Geometry check sheet. Reference: the model listing, model coordinates, mm. Face numbers are marked on the shaded views. A direction names the side the tool comes from. Coordinates: 2 decimals unless noted, no trailing zeros. Write each loop counter-clockwise with the first axis right and the second up, starting at its lowest first coordinate (ties: lowest second). Pieces come first, ordered by that corner, then holes. Notation, with made-up numbers: (33.25, 20) -> (42.25, 20) arc R27 cw to (42.25, 51) -> close; hole circle Ø5 at (74.25, 17.5). An arc over 180 degrees is marked (long way). One line per question, with ' | ' between items.
Autodesk Inventor part; units mm, degrees
ref_plane "YZ Plane" through (0, 0, 0) normal (1, 0, 0) x (0, 1, 0)
ref_plane "XZ Plane" through (0, 0, 0) normal (0, 1, 0) x (-1, 0, 0)
ref_plane "XY Plane" through (0, 0, 0) normal (0, 0, 1) x (1, 0, 0)
sketch "スケッチ1" plane through (0, 0, 0) normal (0, 1, 0) x (-1, 0, 0)
  circle A0 centre (0, 0) radius 27.5
  line L0 (13, 12.85) -> (-13, 12.85)
  line L1 (-13, 12.85) -> (-13, -12.85)
  line L2 (-13, -12.85) -> (13, -12.85)
  line L3 (13, -12.85) -> (13, 12.85)
  circle A1 centre (0, 0) radius 32.5
  circle A2 centre (0, 0) radius 36.5
  line L4 (0, 0) -> (18.4986, -32.0406)
  line L5 (0, 0) -> (31.6099, -18.25)
  line L6 (-13, -12.85) -> (0.651, -36.4942)
  line L7 (13.2, 12.8507) -> (13.2, -12.85)
  line L8 (13.2, -12.85) -> (13, -12.85)
  point P0 (13, 0)
  point P1 (0, 12.85)
  point P2 (13, -34.1065)
  point P3 (-13, -34.1065)
  point P4 (28.1458, -16.25)
  point P5 (13, -7.5056)
  point P6 (18.25, -31.6099)
  point P7 (16.25, -28.1458)
  point P8 (23.8157, -13.75)
  point P9 (-4.7839, -27.0807)
  point P10 (-1.6802, -32.4565)
  point P11 (13.2, -7.621)
  dimension "d0" = 55
  dimension "d1" = 12.85
  dimension "d2" = 26
  dimension "d3" = 5
  dimension "d4" = 4
  dimension "d11" = 60
  dimension "d12" = 30
  dimension "d16" = 0.2
extrude "押し出し1" add sketch "スケッチ1" along normal blind 4 contours L6 L2 L4 A0 | A0 L4 A1 L6 | L5 A1 L4 A0 | A0 L4 L2 L8 L7 L5 | A1 L4 A2 L6 | L5 A2 L4 A1
extrude "押し出し2" add sketch "スケッチ1" along normal blind 9.2 contours A0 L4 A1 L6 | L5 A1 L4 A0
extrude "押し出し3" add sketch "スケッチ1" along normal blind 14.8 contours A1 L4 A2 L6 | L5 A2 L4 A1
chamfer "面取り1" distance 8 angle 45 1 edges at (-18.5312, 0, -31.4459)
sketch "スケッチ2" plane through (-13.2, 0, -12.85) normal (0, 0, 1) x (1, 0, 0)
  circle A0 centre (21.2, 2) radius 0.8
  circle A1 centre (5.2, 2) radius 0.8
  point P0 (13.2, 0)
extrude "押し出し4" cut sketch "スケッチ2" against normal through all
sketch "スケッチ4" plane through (0, 14.8, 0) normal (0, 1, 0) x (1, 0, 0)
  circle A0 centre (-24.3952, 24.3952) radius 0.8
  line L0 (4.7839, 27.0807) -> (-0.651, 36.4942)
  arc A1 (-0.651, 36.4942) -> (-31.6099, 18.25) centre (0, 0) ccw
  line L1 (-31.6099, 18.25) -> (-23.8157, 13.75)
  arc A2 (4.7839, 27.0807) -> (-23.8157, 13.75) centre (0, 0) ccw
  circle A3 centre (-17.25, 29.8779) radius 0.8
  circle A4 centre (-8.9293, 33.3244) radius 0.8
  circle A5 centre (-24.3952, 24.3952) radius 0.8
extrude "押し出し6" cut sketch "スケッチ4" against normal blind 4 contours A0 | A3 | A4
properties part number "waist_side"
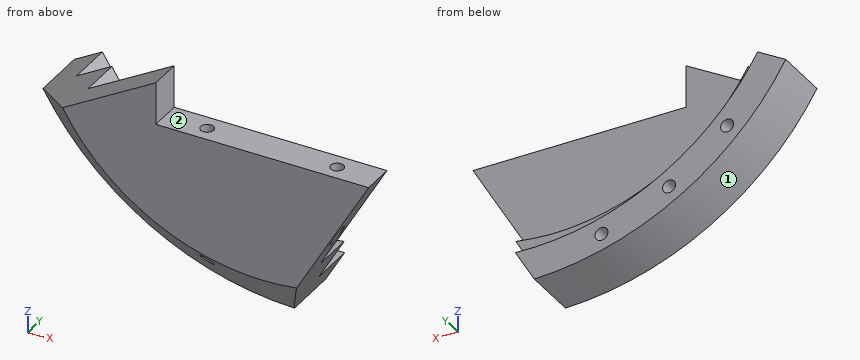
(1) Cross-section at A-A (y = 2). Record the cut outline in (x, z), plus the area to 3 significant figures.
Answers below:
outline: (-26.41, -15.25) arc R30.5 ccw to (-8.8, -29.2) -> (-8.8, -12.85) -> (-13.2, -12.85) -> (-13.2, -7.62) -> close; (-7.2, -29.64) arc R30.5 ccw to (2.89, -30.36) -> (7.2, -22.9) -> (7.2, -12.85) -> (-7.2, -12.85) -> close; (8.8, -20.12) -> (13, -12.85) -> (8.8, -12.85) -> close | area: 467 mm²
(2) Material ranges on line 1 (Y direction, x = -8, z = -21.25); line 2 (Y direction, x = -1, z = -25); line 3 (X direction, y = 7.25, z = -17), recorded low to high.
Answers below:
line 1: y = 0 to 1.2, 2.8 to 4 | line 2: y = 0 to 4 | line 3: x = -29.44 to -21.62
(3) Depth check by flat-ended pin: P1, Ø2, axis at y = 2.5, z = -11, coming from the +X side; P2, Ø10, axis at x = 2, z = -30, coming from the -Y side; P3, Ø5.5, axis at x = -14.5, z = -25.5, coming from the +Y side; P4, Ø1, axis at x = -8, y = 2, coming from the -Z side (1 decimal). Enter the tip coordinate at first touch or a pass-through.
Answers below:
P1: stops at x = -13.2 | P2: stops at y = 0 | P3: stops at y = 9.2 | P4: passes through
(4) Cross-section at B-B (x = 8). Record the cut outline in (y, z).
Answers below:
outline: (0, -21.51) -> (1.2, -21.51) -> (1.2, -12.85) -> (0, -12.85) -> close; (2.8, -21.51) -> (4, -21.51) -> (4, -12.85) -> (2.8, -12.85) -> close
(5) Cross-section at D-D (z = -17). Count the separate pieces of the cut face and the enclosed holes in it, plus the area to 3 significant figures.
Answers below:
separate pieces: 1 | enclosed holes: 2 | area: 189 mm²
(6) Cross-section at C-C (y = 11.75). Record the cut outline in (x, z), plus the area to 3 significant figures.
Answers below:
outline: (-31.61, -18.25) arc R36.5 ccw to (-0.65, -36.49) -> (1.68, -32.46) arc R32.5 cw to (-28.15, -16.25) -> close; hole circle Ø1.6 at (-24.4, -24.4); hole circle Ø1.6 at (-17.25, -29.88); hole circle Ø1.6 at (-8.93, -33.32) | area: 141 mm²
(7) Tool access check on the marked faces 1 and 2. Record the directions out of +Z, -Z, +X, -X, +Y, -Y that give a thin tool (end or side, any length) a straight path to the whole face; none if there is none.
Answers below:
face 1: -Z, -X, +Y, -Y | face 2: +Z, +X, +Y, -Y
